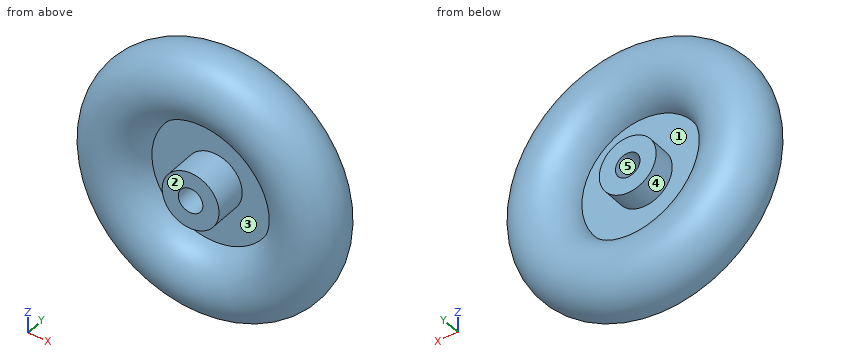
```python
from build123d import *


with BuildPart() as part:
    # 草图1 → 旋转2 (revolve)
    with BuildSketch(Plane.XY, mode=Mode.PRIVATE) as revolve_2_sk:
        with BuildLine():
            Line((15.619751756, 46), (15.619751756, 28.249450756))
            Line((15.619751756, 28.249450756), (41.514974563, 28.249450756))
            ThreePointArc((41.514974563, 28.249450756), (94.514974563, 26.92343472), (41.514974563, 25.597418683))
            Line((41.514974563, 25.597418683), (15.619751756, 25.597418683))
            Line((15.619751756, 25.597418683), (15.619751756, 0))
            Line((15.619751756, 0), (3.119751756, 0))
            Line((3.119751756, 0), (3.119751756, 46))
            Line((3.119751756, 46), (15.619751756, 46))
        make_face()
    revolve(revolve_2_sk.sketch.rotate(Axis((-6.380248244, 0.539107049, 0), (0, 1, 0)), 90), axis=Axis((-6.380248244, 0.539107049, 0), (0, 1, 0)))


solid = part.part
```
Input: part model. Units: mm. Frame: model coordinates. Face numbers are marked on the shaded views. A direction names the side the tool comes from. Round coordinates to 2 decimals unless told otherwise and drop trailing zeros. Order: outer loops, then holes, each group sorted by start corner. A loop starts at its lowest first (then second) coordinate and runs counter-clockwise, first axis right, second up. Notation, with made-up numbers: (83, 56.25) - (111, 56.25) arc R13 ccw to (111, 72.25) - close; hole circle Ø9 at (50, 64.25). An arc over 180 degrees is marked (long way). One line per question, with ' | ' between items. Start each with the question number.
1) Pull-direction query (X, two-part tool) for the marked faces 1 and 2; classes: +X half, -X half, draft (parallel to the pull), parting line (faces both ways), or undercut.
2) Set-up query: the marked faces 3, 4 and 5. Return all of +Z, -Z, +X, -X, +Y, -Y with unobstructed straight access to the full face (end or side cutting, diameter ignored); none if empty.
3) Ray query, probe 1 along Z at (x, y) = (-3, 25); probe 2 along X at (y, z) = (27, 0); probe 3 along X at (y, z) = (31, 0). Return the intervals inside material, ascending.
4) Cut plane C-C, the plane y = 9. Return the cut outline in (x, z).
5) Cut plane B-B, the plane y = 43. Return the cut outline in (x, z), then the cut area to 3 significant figures.
6) Contact query for flat-ended pins moving along their axis: P1, Ø8, axis at y = 44.5, z = 44.5, coming from the +X side; P2, Ø8, axis at x = -36.5, y = 8, coming from the -Z side; P3, Ø10, axis at x = 51, y = 22.5, coming from the +Z side; P4, Ø15, axis at x = -6.38, z = 0, coming from the +Y side. Output: stop coordinate, or through.
7) Cut plane A-A, the plane z = 0. Return the cut outline in (x, y), then the cut area to 3 significant figures.
Worked out:
1) face 1: undercut | face 2: draft
2) face 3: -Y | face 4: +Y | face 5: +Y, -Y
3) probe 1: z = -100.77 to -47.81, -21.74 to -8.88, 8.88 to 21.74, 47.81 to 100.77 | probe 2: x = -107.28 to -15.88, 3.12 to 94.51 | probe 3: x = -106.96 to -54.56, -28.38 to -15.88, 3.12 to 15.62, 41.8 to 94.2
4) outline: circle Ø187.84 at (-6.38, 0); circle Ø44 at (-6.38, 0); hole circle Ø109.67 at (-6.38, 0); hole circle Ø19 at (-6.38, 0)
5) outline: circle Ø190.93 at (-6.38, 0); circle Ø44 at (-6.38, 0); hole circle Ø106.58 at (-6.38, 0); hole circle Ø19 at (-6.38, 0) | area: 20,900 mm^2
6) P1: stops at x = 80.63 | P2: stops at z = -91.74 | P3: stops at z = 85.91 | P4: passes through
7) outline: (-54.28, 25.6) - (-28.38, 25.6) - (-28.38, 0) - (-15.88, 0) - (-15.88, 46) - (-28.38, 46) - (-28.38, 28.25) - (-54.28, 28.25) arc R26.52 ccw (long way) to start; (3.12, 0) - (15.62, 0) - (15.62, 25.6) - (41.51, 25.6) arc R26.52 ccw (long way) to (41.51, 28.25) - (15.62, 28.25) - (15.62, 46) - (3.12, 46) - close | area: 5,710 mm^2
